Part model, mm, in its own coordinate system. Face numbers are marked on the shaded views. A direction names the side the tool comes from. Give positions to 0.01 mm unless a question says otherwise; leave off trailing zeros. Loops run counter-clockwise (first coordinate to the right, second up) from the corner with the lowest first, then second, coordinate; pieces in that order, holes last. Notation, with made-up numbers: (81, -1) -> (98, -1) arc R7 cw to (98, 6) -> close; hole circle Ø11 at (-17.5, 16). An arc over 180 degrees is marked (long way). Write item = value, one per line.
from build123d import *

# Parameters (mm, degrees)
SKETCH_1_R          = 44.5
SKETCH_1_R_2        = 10.9
EXTRUDE_1_DEPTH     = 7
SKETCH_2_R          = 20
SKETCH_2_R_2        = 10.9
EXTRUDE_2_DEPTH     = 15
SKETCH_3_R          = 2
CUT_EXTRUDE_3_DEPTH = 65.695440334
CHAMFER_1_SIZE      = 5


with BuildPart() as part:
    # Эскиз1 → Вытянуть1 (new body)
    with BuildSketch(Plane.XY):
        Circle(SKETCH_1_R)
        Circle(SKETCH_1_R_2, mode=Mode.SUBTRACT)
    extrude(amount=EXTRUDE_1_DEPTH)

    # Эскиз2 → Вытянуть2 (add)
    with BuildSketch(Plane.XY.offset(7)):
        Circle(SKETCH_2_R)
        Circle(SKETCH_2_R_2, mode=Mode.SUBTRACT)
    extrude(amount=EXTRUDE_2_DEPTH)

    # Эскиз3 → Вытянуть3 (cut, through all)
    with BuildSketch(Plane.XY.offset(7)):
        with Locations((0, 35)):
            Circle(SKETCH_3_R)
        with Locations((24.748737342, 24.748737342)):
            Circle(SKETCH_3_R)
        with Locations((35, 0)):
            Circle(SKETCH_3_R)
        with Locations((24.748737342, -24.748737342)):
            Circle(SKETCH_3_R)
        with Locations((0, -35)):
            Circle(SKETCH_3_R)
        with Locations((-24.748737342, -24.748737342)):
            Circle(SKETCH_3_R)
        with Locations((-35, 0)):
            Circle(SKETCH_3_R)
        with Locations((-24.748737342, 24.748737342)):
            Circle(SKETCH_3_R)
    extrude(amount=-CUT_EXTRUDE_3_DEPTH, mode=Mode.SUBTRACT)

    # Фаска1
    chamfer_1_edges = [part.edges().sort_by_distance(p)[0] for p in [
        (-20, 0, 7),
    ]]
    chamfer(chamfer_1_edges, length=CHAMFER_1_SIZE)


solid = part.part
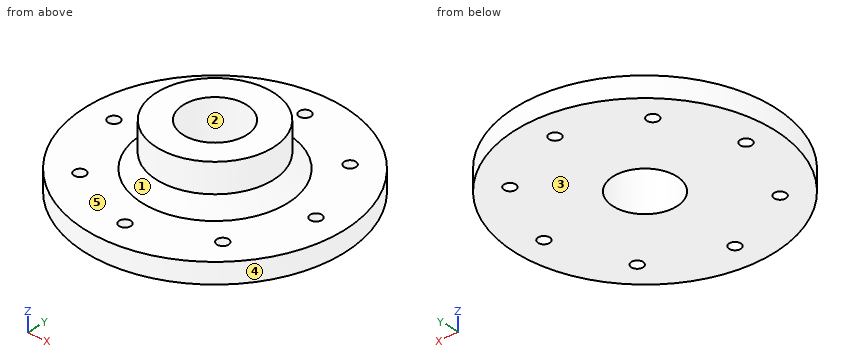
1) Drill centre lines: line 1 along Y through (x, z) = (0, 15); line 2 along Y through (x, z) = (-23.5, 5.5); line 3 along Y through (x, z) = (6, 2). Where is each one in solid material? Low to high. Write a range as [from, to].
Resolved:
line_1 = [-20, -10.9], [10.9, 20]
line_2 = [-37.79, -26.31], [-23.19, 23.19], [26.31, 37.79]
line_3 = [-44.09, -9.1], [9.1, 44.09]
2) Slice it at B-B, the plane y = 35. List the corners of the cut face in (x, z).
Resolved:
outline = (-27.48, 0) -> (-2, 0) -> (-2, 7) -> (-27.48, 7) -> close; (2, 0) -> (27.48, 0) -> (27.48, 7) -> (2, 7) -> close
3) Slice it at A-A, the plane x = 0. List the corners of the cut face in (y, z), and give its area (3 significant figures).
Resolved:
outline = (-44.5, 0) -> (-37, 0) -> (-37, 7) -> (-44.5, 7) -> close; (-33, 0) -> (-10.9, 0) -> (-10.9, 22) -> (-20, 22) -> (-20, 12) -> (-25, 7) -> (-33, 7) -> close; (10.9, 0) -> (33, 0) -> (33, 7) -> (25, 7) -> (20, 12) -> (20, 22) -> (10.9, 22) -> close; (37, 0) -> (44.5, 0) -> (44.5, 7) -> (37, 7) -> close
area = 712 mm²
4) Which spindle directions (+Z, -Z, +X, -X, +Y, -Y) get a long thin tool onto all of the face, cutting with end or side? Do the marked faces 4 and 5. Say none if no direction does.
Resolved:
face_4 = +Z, -Z
face_5 = +Z
5) Drop flat-ended pins along their axis: P1, Ø3, axis at x = 0, y = -35, coming from the +Z side; P2, Ø1, axis at y = -1, z = 15.5, coming from the -X side; P3, Ø4, axis at x = 34, y = -30.5, coming from the +Z side; P4, Ø6, axis at x = -11, z = 4.5, coming from the -Y side (3 decimals). Give the stop position or say it passes through.
Resolved:
P1 = through
P2 = -19.99
P3 = 7
P4 = -43.775
6) Pull direction X, two halves, no side cores. Call the marked faces 1, 2 and 3: pulls with the +X half, pulls with the -X half, needs draft (parallel to the pull), parting line crosses it, or undercut.
Resolved:
face_1 = parting line crosses it
face_2 = undercut
face_3 = needs draft
7) Slice it at D-D, the plane z = 17.25. List the corners of the cut face in (x, y), and give its area (3 significant figures).
Resolved:
outline = circle Ø40 at (0, 0); hole circle Ø21.8 at (0, 0)
area = 883 mm²
